Check sheet for the modelled part. Datum: model origin and axes. Units: mm. A direction names the side the tool comes from. Give positions to 0.01 mm unless a question says otherwise; leave off trailing zeros. Order: outer loops, then holes, each group sorted by start corner. A loop starts at its lowest first (then second) coordinate and runs counter-clockwise, first axis right, second up. Notation, with made-up numbers: M 59.5,74 L 73.5,74 A24 cw 73.5,102 Z; hole C 28,10.5 d8. An arc over 180 degrees is marked long. Return JSON: item names as keys, results as strings. Group by question number.
Autodesk Inventor part; units mm, degrees
ref_plane "YZ Plane" through (0, 0, 0) normal (1, 0, 0) x (0, 1, 0)
ref_plane "XZ Plane" through (0, 0, 0) normal (0, 1, 0) x (-1, 0, 0)
ref_plane "XY Plane" through (0, 0, 0) normal (0, 0, 1) x (1, 0, 0)
sketch "Sketch1" plane through (0, 0, 0) normal (0, 0, 1) x (1, 0, 0)
  line L0 (22.6139, 7.6894) -> (22.6139, 6.2924)
  line L1 (0.7699, 6.2924) -> (0.7699, 7.6894)
  line L2 (11.9459, 3.8794) -> (12.9619, 3.8794)
  line L3 (12.9619, 3.8794) -> (12.9619, 6.2924)
  line L4 (11.9459, 6.2924) -> (11.9459, 3.8794)
  line L5 (11.9459, 6.2924) -> (0.7699, 6.2924)
  line L6 (12.1999, 7.6894) -> (12.1999, 9.7214)
  line L7 (12.1999, 11.1184) -> (12.9619, 11.1184)
  line L8 (12.9619, 11.1184) -> (12.9619, 7.6894)
  line L9 (12.9619, 11.1184) -> (7.8819, 11.1184)
  line L10 (7.8819, 11.1184) -> (7.8819, 9.7214)
  line L11 (7.8819, 9.7214) -> (12.1999, 9.7214)
  line L12 (12.9619, 9.7214) -> (12.9619, 11.1184)
  line L13 (11.9459, 3.8794) -> (0.9057, 3.8794)
  line L14 (0.7699, 7.6894) -> (2.0399, 7.6894)
  line L15 (2.0399, 7.6894) -> (2.0399, 7.3084)
  line L16 (0.7699, 7.6894) -> (2.0399, 7.6894)
  line L17 (7.1199, 7.6894) -> (2.0399, 7.3084)
  line L18 (0.7699, 7.6894) -> (2.0399, 7.6894)
  line L19 (7.1199, 7.6894) -> (12.1999, 7.6894)
  line L20 (18.1054, 7.8164) -> (17.4704, 7.8164)
  line L21 (17.4704, 6.1654) -> (18.1054, 7.8164) construction
  line L22 (18.1054, 6.1654) -> (17.4704, 7.8164) construction
  line L23 (16.8354, 7.8164) -> (16.2004, 7.8164)
  line L24 (16.2004, 6.1654) -> (16.8354, 7.8164) construction
  line L25 (16.8354, 6.1654) -> (16.2004, 7.8164) construction
  line L26 (19.3754, 7.8164) -> (18.7404, 7.8164)
  line L27 (18.7404, 6.1654) -> (19.3754, 7.8164) construction
  line L28 (19.3754, 6.1654) -> (18.7404, 7.8164) construction
  line L29 (16.2004, 7.8164) -> (16.2004, 7.6894)
  line L30 (16.8354, 7.6894) -> (16.8354, 7.8164)
  line L31 (17.4704, 7.8164) -> (17.4704, 7.6894)
  line L32 (18.1054, 7.6894) -> (18.1054, 7.8164)
  line L33 (18.7404, 7.8164) -> (18.7404, 7.6894)
  line L34 (19.3754, 7.6894) -> (19.3754, 7.8164)
  line L35 (19.3265, 7.6894) -> (22.6139, 7.6894)
  line L36 (22.6139, 6.2924) -> (19.3265, 6.2924)
  line L37 (18.0565, 7.6894) -> (18.7892, 7.6894)
  line L38 (12.9619, 7.6894) -> (16.2492, 7.6894)
  line L39 (16.7865, 7.6894) -> (17.5192, 7.6894)
  line L40 (19.3265, 6.2924) -> (16.2492, 6.2924)
  line L41 (16.7865, 6.2924) -> (12.9619, 6.2924)
  point P0 (16.2004, 6.2924)
  point P1 (16.8354, 6.2924)
  point P2 (17.4704, 6.2924)
  point P3 (19.3754, 6.2924)
  dimension "d8" = 21.844
  dimension "d9" = 1.397
  dimension "d10" = 11.176
  dimension "d12" = 11.43
  dimension "d13" = 12.192
  dimension "d15" = 12.192
  dimension "d16" = 7.239
  dimension "d17" = 1.397
  dimension "d18" = 7.112
  dimension "d34" = 1.27
  dimension "d35" = 0.381
  dimension "d36" = 6.35
  dimension "d38" = 0.635
  dimension "d39" = 1.651
  dimension "d41" = 0.635
  dimension "d42" = 1.651
  dimension "d44" = 0.635
  dimension "d45" = 1.651
revolve "Revolution1" add sketch "Sketch1" angle 360 about axis through (11.9459, 3.8794, 0) along (-1, 0, 0)
sketch "Sketch2" plane through (22.6139, 3.8794, 0) normal (1, 0, 0) x (0, 0, -1)
  circle A0 centre (0, 0) radius 3.175
  point P0 (0, -3.8794)
  dimension "d20" = 6.35
extrude "Extrusion1" cut sketch "Sketch2" against normal blind 1.27
sketch "Sketch3" plane through (0.7699, 3.8794, 0) normal (-1, 0, 0) x (0, 0, 1)
  circle A0 centre (0, 0) radius 3.175
  point P0 (0, -3.8794)
  dimension "d26" = 6.35
extrude "Extrusion2" cut sketch "Sketch3" against normal blind 6.35
sketch "Sketch4" plane through (0.7699, 3.8794, 0) normal (-1, 0, 0) x (0, 0, 1)
  line L0 (0.508, -9.525) -> (-0.508, -9.525)
  line L1 (-0.508, -9.525) -> (-0.508, 9.525)
  line L2 (-0.508, 9.525) -> (0.508, 9.525)
  line L3 (0.508, 9.525) -> (0.508, -9.525)
  line L4 (0.508, -9.525) -> (-0.508, 9.525) construction
  line L5 (-0.508, -9.525) -> (0.508, 9.525) construction
  point P0 (0, -3.8794)
  point P1 (0, 0)
  dimension "d30" = 1.016
  dimension "d31" = 19.05
extrude "Extrusion3" cut sketch "Sketch4" against normal blind 5.08
chamfer "Chamfer1" distance 0.127 distance2 0.635 1 edges at (19.3754, -0.0576, 0) measured on face at (19.3754, 7.736, 0.3141)
chamfer "Chamfer2" distance 0.127 distance2 0.635 1 edges at (18.1054, -0.0576, 0) measured on face at (18.1054, 7.736, 0.3141)
chamfer "Chamfer3" distance 0.127 distance2 0.635 1 edges at (16.8354, -0.0576, 0) measured on face at (16.8354, 7.736, 0.3141)
properties part number "Axle"
1) Sectioned sample at C-C on x = 19. Record the boundary of the cut face in (y, z), then the cut area to 3 significant figures.
2) Release check for a two-part mould opening along Z. For faces 5 (the face through (7.882, 4, -6)), 6 (the face through (17.157, 0.856, -2.318)), 7 (the face through (12.962, 4, 0)) record: released by +Z, released by -Z, zero draft, split by the parting line, or undercut.
3) Tool access check on faces 1 (the face through (3.9, 0.78, -0.69)), 2 (the face through (2.04, 3.9, -3.6)), 3 (the face through (0.77, 3.9, 3.4)), 4 (the face through (14.604, 0.856, -2.318)). Record the directions out of +Z, -Z, +X, -X, +Y, -Y that give a thin tool (end or side, any length) a straight path to the whole face; none if there is none.
4) Material ranges on line 1 along Y through (x, z) = (9.1, 0); line 2 along Y through (x, z) = (22, 0); line 3 along Z through (x, y) = (8.5, 2.25), recorded low to high.
5) Sectioned sample at A-A on z = -5.25. Record the boundary of the cut face in (x, y).
6) Depth check by flat-ended pin: P1, Ø1.5, axis at x = 17, y = 5, coming from the -Z side; P2, Ø5.5, axis at y = 3, z = -0.5, coming from the -X side; P3, Ø5.5, axis at y = 3.88, z = 0, coming from the -X side; P4, Ø5, axis at x = 7.5, y = 6.5, coming from the -Z side. Enter the tip coordinate at first touch or a pass-through.
7) Sectioned sample at B-B on y = -1.25. Record the boundary of the cut face in (x, z), then the cut area to 3 significant figures.
Reply:
{
 "1": {"outline": "C 3.88,0 d7.77; hole C 3.88,0 d4.83", "area": "29.1 mm^2"},
 "2": {"face 5": "zero draft", "face 6": "split by the parting line", "face 7": "undercut"},
 "3": {"face 1": "-X", "face 2": "-Z", "face 3": "+Z, -Z, -X, +Y, -Y", "face 4": "none"},
 "4": {"line 1": "-3.36 to -1.96, 0.07 to 1.47, 6.29 to 7.69, 9.72 to 11.12", "line 2": "0.07 to 0.7, 7.05 to 7.69", "line 3": "-7.05 to -5.61, -3.44 to -1.78, 1.78 to 3.44, 5.61 to 7.05"},
 "5": {"outline": "M 7.88,-1.1 L 12.96,-1.1 L 12.96,8.86 L 7.88,8.86 L 7.88,6.44 L 12.2,6.44 L 12.2,1.32 L 7.88,1.32 Z"},
 "6": {"P1": "z = -3.9", "P2": "x = 0.77", "P3": "x = 7.12", "P4": "z = -7.24"},
 "7": {"outline": "M 7.88,-5.11 L 12.96,-5.11 L 12.96,5.11 L 7.88,5.11 L 7.88,2.8 L 12.2,2.8 L 12.2,-2.8 L 7.88,-2.8 Z", "area": "27.8 mm^2"}
}
